Job drawing, mm, ordinate dimensions from the low corner. One solid piece. Give positions to 0.01 mm unless a question says otherwise; leave off trailing zeros. Write each loop counter-clockwise with the first axis right and the second up, starting at its lowest first coordinate (ties: lowest second). Pieces come first, ordered by that corner, then holes. Notation, with made-up numbers: (70.5, 5) -> (75.5, 5) arc R6 cw to (75.5, 15) -> close; hole circle Ø5 at (-17.75, -5.5). An arc over 180 degrees is marked (long way). One line per question, with ' | ' between items. Start each with the question number.
(1) Pin check, flat tips, straight feed: P1, Ø1.5, axis at y = 2, z = 2.5, coming from the +X side; P2, Ø3, axis at y = 1.5, z = 0.5, coming from the +X side. Stop position of each tip, or through.
(2) Band-saw the part on B-B, the plane z = 2. Give the cut face in (x, y) (1 decimal), and give its area (3 significant figures).
(3) Band-saw the part on C-C, the plane y = 3.5. Give the cut face in (x, z).
(4) Band-saw the part on D-D, the plane y = 7.75. Give the cut face in (x, z), and give its area (3 significant figures).
(5) Drill centre lines: probe 1 along X at (y, z) = (4.75, 4.75) (1 decimal); probe 2 along X at (y, z) = (6, 0.75) (1 decimal); probe 3 along Y at (x, z) = (5, 4) (1 decimal). Where is each one in solid material? Low to high. Write a range as from..to.
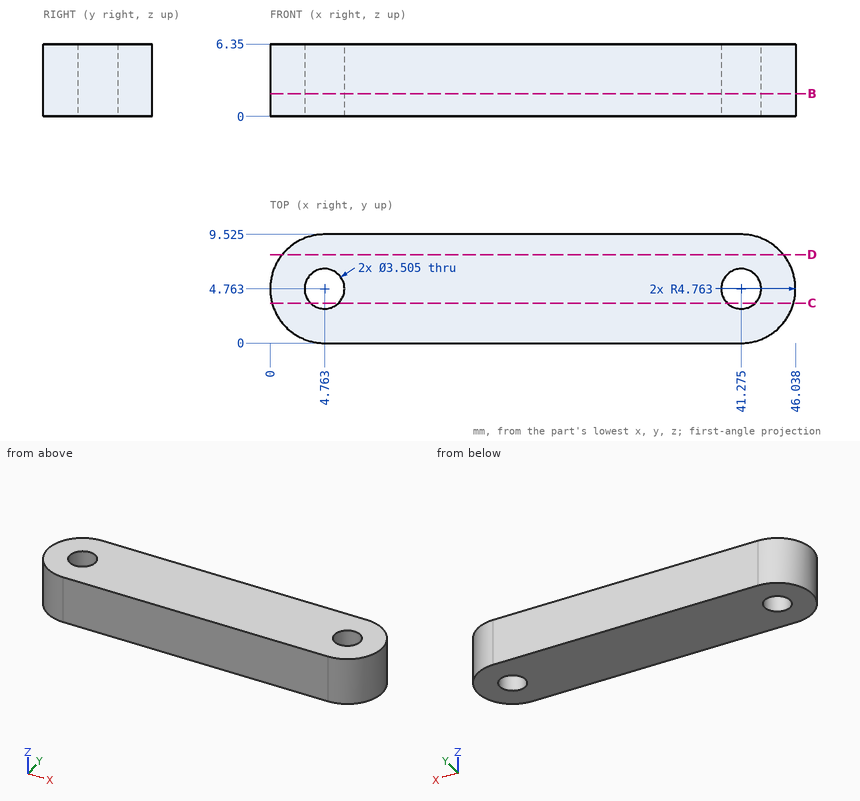
Results:
1) P1: stops at x = 45.59 | P2: stops at x = 45.7
2) outline: (4.8, 0) -> (41.3, 0) arc R4.8 ccw to (41.3, 9.5) -> (4.8, 9.5) arc R4.8 ccw to start; hole circle Ø3.5 at (4.8, 4.8); hole circle Ø3.5 at (41.3, 4.8) | area: 400 mm²
3) outline: (0.17, 0) -> (3.55, 0) -> (3.55, 6.35) -> (0.17, 6.35) -> close; (5.98, 0) -> (40.06, 0) -> (40.06, 6.35) -> (5.98, 6.35) -> close; (42.49, 0) -> (45.87, 0) -> (45.87, 6.35) -> (42.49, 6.35) -> close
4) outline: (1.05, 0) -> (44.98, 0) -> (44.98, 6.35) -> (1.05, 6.35) -> close | area: 279 mm²
5) probe 1: x = 0..3, 6.5..39.5, 43..46 | probe 2: x = 0.2..3.5, 6..40, 42.5..45.9 | probe 3: y = 0..3, 6.5..9.5
